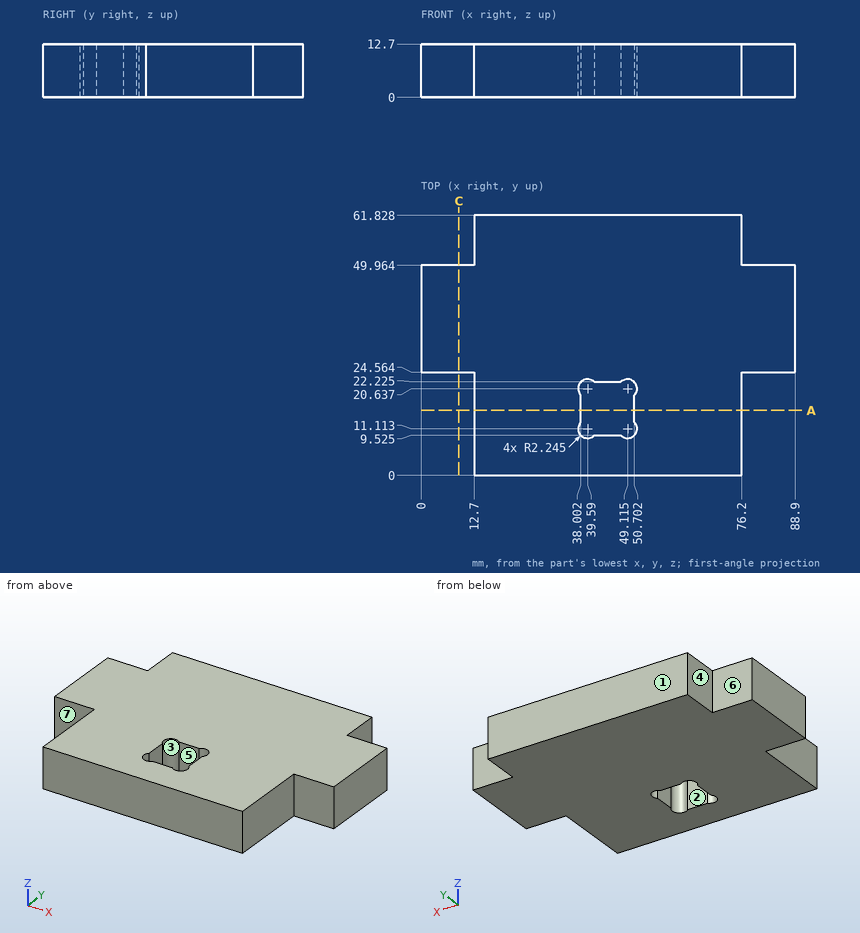
Job drawing, mm, ordinate dimensions from the low corner. One solid piece. A direction names the side the tool comes from. Give positions to 0.01 mm unless a question says otherwise; leave off trailing zeros. Write each loop counter-clockwise with the first axis right and the second up, starting at its lowest first coordinate (ties: lowest second). Pieces come first, ordered by that corner, then holes. Notation, with made-up numbers: M -10.5,16 L 43.5,16 A22 cw 43.5,25 Z; hole C 15,-33 d3. An arc over 180 degrees is marked long. One line per item, written item: value. Start each with the question number.
Q1. Probe probe 1 along X at (y, z) = (16, 0.5); probe 2 along X at (y, z) = (23, 6.75); probe 3 along X at (y, z) = (11.5, 8.5) (1 decimal). List the from-to ranges inside material, lowest first. Write a range as [from, to].
Q2. Two-plate mould, pull along X, no slides. Class the marked faces 1, 2, 3 and 4: +X half, -X half, draft (parallel to the pull), parting line (faces both ways), or undercut.
Q3. Drop flat-ended pins along their axis: pin 1 Ø6 at (y, z) = (56, 6.5) entering from +X; pin 2 Ø6 at (x, y) = (47, 21.5) entering from -Z; pin 3 Ø1.9 at (y, z) = (14.5, 4.5) entering from -X; pin 4 Ø4 at (x, z) = (85, 8) entering from -Y. Give the stop position or say it passes through.
Q4. Saw through at A-A, the plane y = 15.5. Write the cut outline in (x, z).
Q5. 3-axis set-ups, long thin cutter, end or side, ignore diameter. For the marked faces 5, 6 and 7: which of +Z, -Z, +X, -X, +Y, -Y reach the whole face in a straight line?
Q6. Saw through at C-C, the plane x = 9. Write the cut outline in (y, z), plus the area to 3 significant figures.
Output values:
1. probe 1: x = [12.7, 38], [50.7, 76.2]
1. probe 2: x = [12.7, 76.2]
1. probe 3: x = [12.7, 37.4], [51.3, 76.2]
2. face 1: draft
2. face 2: undercut
2. face 3: undercut
2. face 4: -X half
3. pin 1: stops at x = 76.2
3. pin 2: stops at z = 0
3. pin 3: stops at x = 12.7
3. pin 4: stops at y = 24.56
4. outline: M 12.7,0 L 38,0 L 38,12.7 L 12.7,12.7 Z; M 50.7,0 L 76.2,0 L 76.2,12.7 L 50.7,12.7 Z
5. face 5: +Z, -Z
5. face 6: +Z, -Z, -X, +Y
5. face 7: +Z, -Z, -X, -Y
6. outline: M 24.56,0 L 49.96,0 L 49.96,12.7 L 24.56,12.7 Z
6. area: 323 mm²
